```python
from build123d import *

# Parameters (mm, degrees)
SKETCH1_W           = 152.4
SKETCH1_H           = 43.942
BOSS_EXTRUDE1_DEPTH = 10.16
SKETCH2_W           = 139.7
SKETCH2_H           = 33.782
SKETCH2_W_2         = 6.35
CUT_EXTRUDE1_DEPTH  = 8.89
CHAMFER1_SIZE       = 5.08
FILLET1_R           = 12.7
FILLET2_R           = 1.27


# Some blends are built 0.0001 mm under size
with BuildPart() as part:
    # Sketch1 → Boss-Extrude1 (new body)
    with BuildSketch(Plane(origin=(0, 0, 0), x_dir=(1, 0, 0), z_dir=(0, 1, 0))):
        Rectangle(SKETCH1_W, SKETCH1_H)
    extrude(amount=BOSS_EXTRUDE1_DEPTH)

    # Sketch2 → Cut-Extrude1 (cut)
    with BuildSketch(Plane(origin=(0, 10.16, 0), x_dir=(1, 0, 0), z_dir=(0, 1, 0))):
        Rectangle(SKETCH2_W, SKETCH2_H)
        with Locations((73.025, 0)):
            Rectangle(SKETCH2_W_2, SKETCH2_H)
        with Locations((-73.025, 0)):
            Rectangle(SKETCH2_W_2, SKETCH2_H)
    extrude(amount=-CUT_EXTRUDE1_DEPTH, mode=Mode.SUBTRACT)

    # Chamfer1
    chamfer1_edges = [part.edges().sort_by_distance(p)[0] for p in [
        (0, 10.16, 16.891),
        (0, 10.16, -16.891),
    ]]
    chamfer(chamfer1_edges, length=CHAMFER1_SIZE - 0.0001)  # a hair under: the kernel refuses the full size

    # Fillet1
    # the kernel refuses this fillet: 12.7 mm, written as the material it takes off along each edge
    with BuildSketch(Plane(origin=(89.017910379, 5.0801, 16.891), x_dir=(0, -1, 0), z_dir=(-1, 0, 0))) as fillet1_piece_1:
        with BuildLine():
            CenterArc((5.354803581, 12.605708661), FILLET1_R, 225, 38.013804416)
            Line((-3.62545254, 3.62545254), (-3.805057662, 3.445847418))
            Line((-3.805057662, 3.445847418), (-0.179605122, -0.179605122))
            Line((-0.179605122, -0.179605122), (0, -0.254))
            ThreePointArc((0, -0.254), (1.90505, -0.254), (3.779205928, -0.252114173))
            Line((3.779205928, -0.252114173), (3.8101, 0))
        make_face()
    extrude(amount=178.035820759, mode=Mode.SUBTRACT)
    with BuildSketch(Plane(origin=(89.017910379, 5.0801, -16.891), x_dir=(0, 0.7071067811865476, -0.7071067811865476), z_dir=(-1, 0, 0))) as fillet1_piece_2:
        with BuildLine():
            CenterArc((5.127164152, 12.7), FILLET1_R, 231.986195584, 38.013804416)
            Line((-2.694147547, 2.694147547), (-2.850573781, 2.494030498))
            ThreePointArc((-2.850573781, 2.494030498), (-1.526678896, 1.167468651), (-0.179605122, -0.179605122))
            Line((-0.179605122, -0.179605122), (0, -0.254))
            Line((0, -0.254), (5.127164152, -0.254))
            Line((5.127164152, -0.254), (5.127164152, 0))
        make_face()
    extrude(amount=178.035820759, mode=Mode.SUBTRACT)

    # Fillet2
    fillet2_edges = [part.edges().sort_by_distance(p)[0] for p in [
        (0, 1.27, 16.891),
        (0, 1.27, -16.891),
    ]]
    fillet(fillet2_edges, radius=FILLET2_R)


solid = part.part
```
Design review of the part built by this model. Coordinates are the model's own, in mm. A direction names the side the tool comes from. Coordinates: 2 decimals unless noted, no trailing zeros. Order: outer loops, then holes, each group sorted by start corner. A loop starts at its lowest first (then second) coordinate and runs counter-clockwise, first axis right, second up.
1) For faces 1 (the cylindrical face through (1.07, 5.79, 18.34)), 2 (the flat face through (76.2, 1, 0)), list the 3-axis set-ups (+Z, -Z, +X, -X, +Y, -Y) from which the entire face can be reached by the end or side of a thin tool; tool diameter is ignored.
2) Clearance check with a flat-ended pin moving along its axis: pin 1 (9.5 mm diameter, centred on x = -23.5, z = -3, fed in from +Y). State where the tip first meets the part, or that it passes through.
3) Take a section at C-C, the plane z = 6.5. Give the boundary of the cut face in (x, y), and give its area (3 significant figures).
4) Take a section at A-A, the plane y = 4.5. Give the boundary of the cut face in (x, z), and give its area (3 significant figures).
5) Mouldability with a two-part tool opening along Z and no side actions: class faces 3 (the flat face through (-76.2, 1, 0)), 4 (the flat face through (-1, 5, 21.971)), 5 (the cylindrical face through (1.07, 5.7, -18.29)) as +Z half, -Z half, draft (parallel to the pull), parting line (faces both ways), or undercut.
6) Wall thickness on line 1 along Y through (x, z) = (55.5, 13.5); line 2 along Z through (x, y) = (8, 6.5); line 3 along Z through (x, y) = (-5, 3.5): over which ranges is each line inside the solid? List them lowest first.
Returned:
1. face 1: +X, -X, +Y
1. face 2: +Z, -Z, +X, +Y, -Y
2. pin 1: stops at y = 1.27
3. outline: (-76.2, 0) - (76.2, 0) - (76.2, 1.27) - (-76.2, 1.27) - close
3. area: 194 mm2
4. outline: (-76.2, -21.97) - (76.2, -21.97) - (76.2, -17.73) - (-76.2, -17.73) - close; (-76.2, 17.73) - (76.2, 17.73) - (76.2, 21.97) - (-76.2, 21.97) - close
4. area: 1,290 mm2
5. face 3: draft
5. face 4: +Z half
5. face 5: undercut
6. line 1: y = 0 to 1.27
6. line 2: z = -21.97 to -18.75, 18.75 to 21.97
6. line 3: z = -21.97 to -17.37, 17.37 to 21.97
